from build123d import *

# Parameters (mm, degrees)
SKETCH2_W                      = 113
SKETCH2_H                      = 104
TOP_FACE_DEPTH                 = 10
SKETCH3_R                      = 3.25
CUT_EXTRUDE1_DEPTH             = 10
CUT_EXTRUDE2_DEPTH             = 10
FILLET1_R                      = 5
CBORE_FOR_M4_SHCS1_D           = 4.8
CBORE_FOR_M4_SHCS1_CBORE_D     = 8
CBORE_FOR_M4_SHCS1_CBORE_DEPTH = 4


with BuildPart() as part:
    # Sketch2 → Top Face (new body)
    with BuildSketch(Plane(origin=(0, 0, 0), x_dir=(1, 0, 0), z_dir=(0, 1, 0))):
        with Locations((0, 12.5)):
            Rectangle(SKETCH2_W, SKETCH2_H)
    extrude(amount=TOP_FACE_DEPTH)

    # Sketch3 → Cut-Extrude1 (cut)
    with BuildSketch(Plane.XZ):
        with Locations(Location((-29, 25, 0), (0, 0, 270))):
            Circle(SKETCH3_R)
        with Locations(Location((-29, -25, 0), (0, 0, 270))):
            Circle(SKETCH3_R)
        with Locations(Location((29, -25, 0), (0, 0, 270))):
            Circle(SKETCH3_R)
        with Locations(Location((29, 25, 0), (0, 0, 270))):
            Circle(SKETCH3_R)
    extrude(amount=-CUT_EXTRUDE1_DEPTH, mode=Mode.SUBTRACT)

    # Sketch4 → Cut-Extrude2 (cut)
    with BuildSketch(Plane(origin=(0, 10, 0), x_dir=(1, 0, 0), z_dir=(0, 1, 0))):
        Polygon((0, 34.5), (-41.5, 0), (0, -34.5), (41.5, 0), align=None)
    extrude(amount=-CUT_EXTRUDE2_DEPTH, mode=Mode.SUBTRACT)

    # Fillet1
    fillet1_edges = [part.edges().sort_by_distance(p)[0] for p in [
        (0, 5, -34.5),
        (41.5, 5, 0),
        (0, 5, 34.5),
        (-41.5, 5, 0),
    ]]
    fillet(fillet1_edges, radius=FILLET1_R)

    # CBORE for M4 SHCS1 (through all)
    with Locations(Plane(origin=(0, 10, 0), x_dir=(1, 0, 0), z_dir=(0, 1, 0))):
        with Locations((47.5, 44.5), (47.5, 24.5), (-47.5, 24.5), (-47.5, 44.5)):
            CounterBoreHole(CBORE_FOR_M4_SHCS1_D / 2, CBORE_FOR_M4_SHCS1_CBORE_D / 2, CBORE_FOR_M4_SHCS1_CBORE_DEPTH)


solid = part.part
Work out the finished part from the listing and answer in its coordinate system (mm). A direction names the side the tool comes from. Give positions to 0.01 mm unless a question says otherwise; leave off trailing zeros. Order: outer loops, then holes, each group sorted by start corner. A loop starts at its lowest first (then second) coordinate and runs counter-clockwise, first axis right, second up. Notation, with made-up numbers: (83, -23) -> (128, -23) arc R8 ccw to (128, -9) -> close; hole circle Ø4 at (19, 38.25). An arc over 180 degrees is marked (long way). One line per item, written item: value.
Item 1: Straight lines are drawn through the part: probe 1 along Z at (x, y) = (47.5, 8.6); probe 2 along Z at (x, y) = (47.5, 1.75); probe 3 along X at (y, z) = (8, -44.5). For each, find the intervals that lie inside material, in ascending order.
Answer sheet:
probe 1: -64.5 to -48.5, -40.5 to -28.5, -20.5 to 39.5
probe 2: -64.5 to -46.9, -42.1 to -26.9, -22.1 to 39.5
probe 3: -56.5 to -51.5, -43.5 to 43.5, 51.5 to 56.5
Item 2: Find section A-A, the plane x = -47.5. Give the vertices of the cut face in (y, z).
Answer sheet:
outline: (0, -64.5) -> (10, -64.5) -> (10, -48.5) -> (6, -48.5) -> (6, -46.9) -> (0, -46.9) -> close; (0, -42.1) -> (6, -42.1) -> (6, -40.5) -> (10, -40.5) -> (10, -28.5) -> (6, -28.5) -> (6, -26.9) -> (0, -26.9) -> close; (0, -22.1) -> (6, -22.1) -> (6, -20.5) -> (10, -20.5) -> (10, 39.5) -> (0, 39.5) -> close
Item 3: Find section C-C, the plane z = -44.5. Give the vertices of the cut face in (x, y).
Answer sheet:
outline: (-56.5, 0) -> (-49.9, 0) -> (-49.9, 6) -> (-51.5, 6) -> (-51.5, 10) -> (-56.5, 10) -> close; (-45.1, 0) -> (45.1, 0) -> (45.1, 6) -> (43.5, 6) -> (43.5, 10) -> (-43.5, 10) -> (-43.5, 6) -> (-45.1, 6) -> close; (49.9, 0) -> (56.5, 0) -> (56.5, 10) -> (51.5, 10) -> (51.5, 6) -> (49.9, 6) -> close
Item 4: Find section B-B, the plane y = 4.75. State how many separate pieces and enclosed holes the cut face has, plus the area to 3 significant figures.
Answer sheet:
separate pieces: 1
enclosed holes: 9
area: 8,710 mm²
Item 5: A flat-ended cylindrical pin translates along its axis: P1, Ø6.5, axis at x = -47, z = -24.5, coming from the +Y side. Find the tip coordinate at first contact, or state that the pin passes through.
Answer sheet:
P1: y = 6
Item 6: A tool of negligible diameter and unlimited length cuts with its end or side. For faces 1 (the flat face through (50.1, 6, -44.6)), 2 (the flat face through (-13, 0, -25)), 3 (the flat face through (19.8, 5.07, 18.04)), from which of +Z, -Z, +X, -X, +Y, -Y can it reach the whole face along a straight path? Write none if from no direction.
Answer sheet:
face 1: +Y
face 2: +Z, -Z, +X, -X, -Y
face 3: +Y, -Y
Item 7: Find section D-D, the plane z = -19. Give the vertices of the cut face in (x, y), plus the area to 3 significant figures.
Answer sheet:
outline: (-56.5, 0) -> (-18.64, 0) -> (-18.64, 10) -> (-56.5, 10) -> close; (18.64, 0) -> (56.5, 0) -> (56.5, 10) -> (18.64, 10) -> close
area: 757 mm²
Item 8: Determine the mould class of faces 4 (the flat face through (-1, 5, -64.5)), 5 (the flat face through (56.5, 5, -12)), 6 (the cylindrical face through (-32.173, 4.93, -24.295)), 7 (the cylindrical face through (25.827, 4.93, -24.295)) for opening direction X: released by +X, released by -X, zero draft, split by the parting line, or undercut.
Answer sheet:
face 4: zero draft
face 5: released by +X
face 6: undercut
face 7: undercut
